Verification items for the finished model (mm, model axes). A direction names the side the tool comes from. Coordinates: 2 decimals unless noted, no trailing zeros. Order: outer loops, then holes, each group sorted by start corner. A loop starts at its lowest first (then second) coordinate and runs counter-clockwise, first axis right, second up. Notation, with made-up numbers: M 56,83 L 77,83 A30 ccw 77,121 Z; hole C -27.5,9.5 d11. An arc over 180 degrees is marked long. Answer as a JSON object with one key per item and string values. Group by question number.
(1) Cross-section at A-A (y = -301.5). Enter the section's corners in (x, z), plus the area to 3 significant figures.
(2) Access from +Z, -Z, +X, -X, +Y, -Y to the whole of each face (thin tool, end or side, straight path). Record for faces 5 (the face through (195.53, -704, -724)), 6 (the face through (-180.14, -112.7, 74.14)), 7 (the face through (957.53, -191, -382)), 8 (the face through (487, -812, 130.759)).
(3) Cross-section at D-D (x = 258). Enter the section's corners in (y, z), plus the area to 3 significant figures.
(4) Cross-section at B-B (z = -289). Enter the section's corners in (x, y).
(5) Mould release check, pull along X, two halves, no side actions. Record for faces 1 (the face through (601.33, -433.42, 226.32)), 2 (the face through (-566.47, -113, 67)), 3 (the face through (571, -1193.8, -721)), 4 (the face through (-1328.47, -113, -239)): released by +X, released by -X, zero draft, split by the parting line, or undercut.
(6) Cross-section at C-C (y = -622.3). Enter the section's corners in (x, z), plus the area to 3 significant figures.
(7) Gauge pin test, flat end, axial feed: pin 1 Ø8 at (x, z) = (-845, -674.5) entering from -Y. Record the tip position at first contact, or that the pin passes through.
(8) Material ranges on line 1 (X direction, y = -917.5, z = 191); line 2 (Y direction, x = -208.5, z = -269); line 3 (X direction, y = -212, z = -280), recorded low to high.
from build123d import *

# Parameters (mm, degrees)
F1_DEPTH       = 25.4
F2_DEPTH       = 203.2
F3_W           = 762
F3_H           = 193.8281174898
F3_H_2         = 191.8793287277
F4_DEPTH       = 965.2
F7_D           = 381
F7_DEPTH       = 203.2
F7_TIP         = 114.4639479248
F7_ON_F6_D     = 381
F7_ON_F6_DEPTH = 203.2
F7_ON_F6_TIP   = 114.4639479248
F9_D           = 381
F9_DEPTH       = 381
F9_TIP         = 114.4639479248


with BuildPart() as f1:
    # F0 (on Front) → F1 (new body)
    with BuildSketch(Plane.XZ):
        Polygon((-566.4698105954, 324.5866265297), (-1328.4698105954, 324.5866265297), (-1328.4698105954, -818.4133734703), (957.5301894046, -818.4133734703), (957.5301894046, 324.5866265297), (195.5301894046, 324.5866265297), (-566.4698105954, -183.4133734703), align=None)
    extrude(amount=F1_DEPTH)

    # F2 (add): a face of the model
    f2_faces = [f1.faces().sort_by_distance(p)[0] for p in [
        (-175.3098105954, -25.4, -279.0867068036),
    ]]
    extrude(f2_faces, amount=F2_DEPTH)

    # F3 (on face) → F4 (join)
    with BuildSketch(Plane.XZ.offset(228.6)):
        with Locations((576.5301894046, 227.6725677848)):
            Rectangle(F3_W, F3_H)
        with Locations((576.5301894046, -722.4737091064)):
            Rectangle(F3_W, F3_H_2)
    extrude(amount=F4_DEPTH)

    # F7
    with Locations(Plane.XY.offset(324.5866265297)):
        with Locations((576.5301894046, -622.3)):
            Hole(F7_D / 2, depth=F7_DEPTH)
            with Locations((0, 0, -(F7_DEPTH + F7_TIP / 2))):  # 118° drill point
                Cone(0, F7_D / 2, F7_TIP, mode=Mode.SUBTRACT)

    # F7 on F6 (one way)
    with BuildSketch(Plane.XY.offset(-626.5340447426)):
        with Locations((576.5301894046, -622.3)):
            Circle(F7_ON_F6_D / 2)
    extrude(amount=-F7_ON_F6_DEPTH, mode=Mode.SUBTRACT)
    with Locations(Plane.XY.offset(-626.5340447426)):
        with Locations((576.5301894046, -622.3)):
            with Locations((0, 0, -(F7_ON_F6_DEPTH + F7_ON_F6_TIP / 2))):  # 118° drill point
                Cone(0, F7_ON_F6_D / 2, F7_ON_F6_TIP, mode=Mode.SUBTRACT)

    # F9
    with Locations(Plane.XZ.offset(228.6)):
        with Locations((-947.4698105954, -246.9133734703)):
            Hole(F9_D / 2, depth=F9_DEPTH)
            with Locations((0, 0, -(F9_DEPTH + F9_TIP / 2))):  # 118° drill point
                Cone(0, F9_D / 2, F9_TIP, mode=Mode.SUBTRACT)


solid = f1.part
Taken from the geometry:
{
 "1": {"outline": "M 195.53,-818.41 L 957.53,-818.41 L 957.53,-626.53 L 195.53,-626.53 Z; M 195.53,130.76 L 957.53,130.76 L 957.53,324.59 L 195.53,324.59 Z", "area": "294,000 mm²"},
 "2": {"face 5": "+Z, -Z, -X, -Y", "face 6": "+Z, +Y, -Y", "face 7": "+Z, -Z, +X, +Y, -Y", "face 8": "+X, -X, -Y"},
 "3": {"outline": "M -1193.8,-818.41 L 0,-818.41 L 0,324.59 L -1193.8,324.59 L -1193.8,130.76 L -228.6,130.76 L -228.6,-626.53 L -1193.8,-626.53 Z", "area": "634,000 mm²"},
 "4": {"outline": "M -1328.47,-228.6 L -1133.26,-228.6 L -1133.26,0 L -1328.47,0 Z; M -761.68,-228.6 L 957.53,-228.6 L 957.53,0 L -761.68,0 Z"},
 "5": {"face 1": "undercut", "face 2": "undercut", "face 3": "zero draft", "face 4": "released by -X"},
 "6": {"outline": "M 195.53,-818.41 L 386.03,-818.41 L 386.03,-626.53 L 195.53,-626.53 Z; M 195.53,130.76 L 386.03,130.76 L 386.03,324.59 L 195.53,324.59 Z; M 767.03,-818.41 L 957.53,-818.41 L 957.53,-626.53 L 767.03,-626.53 Z; M 767.03,130.76 L 957.53,130.76 L 957.53,324.59 L 767.03,324.59 Z", "area": "147,000 mm²"},
 "7": {"pin 1": "stops at y = -228.6"},
 "8": {"line 1": "x = 195.53 to 957.53", "line 2": "y = -228.6 to 0", "line 3": "x = -1328.47 to -1135.07, -759.87 to 957.53"}
}
